For this review, use the dimensioned drawing (mm, ordinates from the lowest corner) and the shaded views. A direction names the side the tool comes from. Give positions to 0.01 mm unless a question says otherwise; leave off trailing zeros. Order: outer loops, then holes, each group sorted by start corner. A loop starts at its lowest first (then second) coordinate and runs counter-clockwise, first axis right, second up.
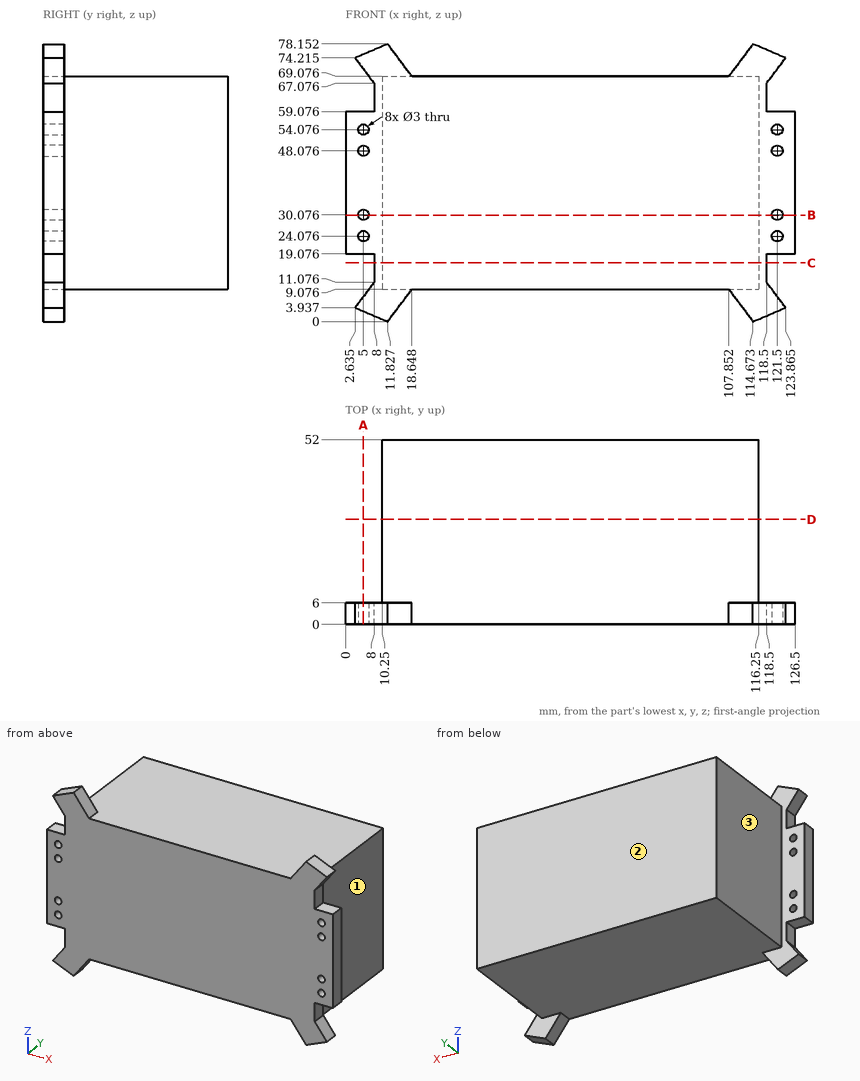
1. Take a section at D-D (y = 29.5). State the section outline as (x, z) points, then the cut area to 3 significant figures.
Recorded:
outline: (10.25, 9.08) - (116.25, 9.08) - (116.25, 69.08) - (10.25, 69.08) - close
area: 6,360 mm2
2. Take a section at B-B (z = 30). State the section outline as (x, y) points.
Recorded:
outline: (0, 0) - (3.5, 0) - (3.5, 6) - (0, 6) - close; (6.5, 0) - (120, 0) - (120, 6) - (116.25, 6) - (116.25, 52) - (10.25, 52) - (10.25, 6) - (6.5, 6) - close; (123, 0) - (126.5, 0) - (126.5, 6) - (123, 6) - close
3. Machinability: for the marked faces 1, 2 and 3, which of the approach directions +Z, -Z, +X, -X, +Y, -Y give a long, thin tool a straight path to every point of the face, cutting with its end or side? Answer none if there is none.
Recorded:
face 1: +Z, -Z, +X, +Y
face 2: +Z, -Z, +X, -X, +Y
face 3: +Z, -Z, -X, +Y
4. For line 1 along X through (y, z) = (41, 37.5); line 2 along Z through (x, y) = (113, 42); line 3 along X through (y, z) = (3, 62), list the stretches that pass through material, from the lowest coordinate up.
Recorded:
line 1: x = 10.25 to 116.25
line 2: z = 9.08 to 69.08
line 3: x = 8 to 118.5
5. Take a section at A-A (x = 5). State the section outline as (y, z) points (1 decimal), then the cut area to 3 significant figures.
Recorded:
outline: (0, 2.9) - (6, 2.9) - (6, 7.1) - (0, 7.1) - close; (0, 19.1) - (6, 19.1) - (6, 22.6) - (0, 22.6) - close; (0, 25.6) - (6, 25.6) - (6, 28.6) - (0, 28.6) - close; (0, 31.6) - (6, 31.6) - (6, 46.6) - (0, 46.6) - close; (0, 49.6) - (6, 49.6) - (6, 52.6) - (0, 52.6) - close; (0, 55.6) - (6, 55.6) - (6, 59.1) - (0, 59.1) - close; (0, 71.1) - (6, 71.1) - (6, 75.2) - (0, 75.2) - close
area: 218 mm2
6. Take a section at C-C (z = 16.5). State the section outline as (x, y) points.
Recorded:
outline: (8, 0) - (118.5, 0) - (118.5, 6) - (116.25, 6) - (116.25, 52) - (10.25, 52) - (10.25, 6) - (8, 6) - close
7. For pin 1 (1 mm diameter, centred on y = 18, z = 46.5, fed in from -X); pin 2 (5 mm diameter, centred on x = 121.5, z = 24.08, fed in from +Y); pin 3 (3 mm diameter, centred on y = 4.5, z = 15, fed in from +X), all flat-tipped, find the tip position at first contact; note any pin that passes through.
Recorded:
pin 1: stops at x = 10.25
pin 2: stops at y = 6
pin 3: stops at x = 118.5
